Geometry: final body of the model. Coordinates: model frame, mm. Coordinates: 2 decimals unless noted, no trailing zeros. Order: outer loops, then holes, each group sorted by start corner. A loop starts at its lowest first (then second) coordinate and runs counter-clockwise, first axis right, second up. Notation, with made-up numbers: (31.5, 12.25) - (36.5, 12.25) arc R26 cw to (36.5, 35.25) - close; hole circle Ø9 at (53, 53.5). An arc over 180 degrees is marked (long way). Use a Markdown table: item, result. Add a question column.
```python
from build123d import *

# Parameters (mm, degrees)
SKETCH1_R           = 31.75
BOSS_EXTRUDE1_DEPTH = 19.05
CUT_EXTRUDE1_DEPTH  = 5.08
CIRPATTERN1_COUNT   = 24


with BuildPart() as part:
    # Sketch1 → Boss-Extrude1 (new body)
    with BuildSketch(Plane(origin=(0, 0, 0), x_dir=(1, 0, 0), z_dir=(0, 1, 0))):
        Circle(SKETCH1_R)
    extrude(amount=BOSS_EXTRUDE1_DEPTH)

    # Sketch2 → Cut-Extrude1 (cut)
    with BuildSketch(Plane(origin=(0, 19.05, 0), x_dir=(1, 0, 0), z_dir=(0, 1, 0))):
        with BuildLine():
            Line((0.431861346, 25.396328392), (0.481566937, 29.206030084))
            ThreePointArc((0.481566937, 29.206030084), (-2.110193645, 29.133677811), (-4.685328245, 28.831784531))
            Line((-4.685328245, 28.831784531), (-4.021364533, 25.079645677))
            ThreePointArc((-4.021364533, 25.079645677), (-1.801722861, 25.336017736), (0.431861346, 25.396328392))
        make_face()
    cut_extrude1 = extrude(amount=-CUT_EXTRUDE1_DEPTH, mode=Mode.SUBTRACT)

    # CirPattern1: Cut-Extrude1 ×24 about axis
    cirpattern1_axis = Axis((0, 0, 0), (0, 1, 0))
    for i in range(1, CIRPATTERN1_COUNT):
        add(cut_extrude1.rotate(cirpattern1_axis, i * 360 / CIRPATTERN1_COUNT), mode=Mode.SUBTRACT)


solid = part.part
```
1) Pin query (flat end, axial travel): pin 1 (6 mm diameter, centred on x = -18, y = 10.5, fed in from -Z); pin 2 (6.5 mm diameter, centred on x = -19.5, z = 20, fed in from +Y); pin 3 (5 mm diameter, centred on x = -15, y = 13, fed in from +Z); pin 4 (3 mm diameter, centred on y = 7, z = -13, fed in from +X). Return the tip coordinate at first contact, or that it passes through.
2) Ray query, line 1 along X through (y, z) = (14, 17.5); line 2 along X through (y, z) = (17, -20); line 3 along Y through (x, z) = (13.5, 24). Return the intervals inside material, ascending.
3) Section A-A (y = 12.25). Return loops of the section in (x, z).
Values follow:
| question | item | result |
|---|---|---|
| 1 | pin 1 | stops at z = -27.98 |
| 1 | pin 2 | stops at y = 19.05 |
| 1 | pin 3 | stops at z = 29.19 |
| 1 | pin 4 | stops at x = 29.59 |
| 2 | line 1 | x = -26.49 to -23.39, -21.47 to 18.41, 23.39 to 26.49 |
| 2 | line 2 | x = -24.66 to -21.29, -19.34 to -16.27, -15.66 to 15.66, 20.67 to 24.66 |
| 2 | line 3 | y = 0 to 13.97 |
| 3 | outline | circle Ø63.5 at (0, 0) |
